Verification items for the finished model (mm, model axes). Face numbers are marked on the shaded views. A direction names the side the tool comes from. Give positions to 0.01 mm unless a question says otherwise; leave off trailing zeros. Order: outer loops, then holes, each group sorted by start corner. A loop starts at its lowest first (then second) coordinate and runs counter-clockwise, first axis right, second up. Notation, with made-up numbers: M -29,3.25 L 15,3.25 A11 ccw 15,7.25 Z; hole C 3,53.25 d4. An arc over 180 degrees is marked long. Answer as a JSON object with one key per item and string values.
```python
from build123d import *

# Parameters (mm, degrees)
CROQUIS1_W              = 100
CROQUIS1_H              = 42
SALIENTE_EXTRUIR1_DEPTH = 5
CROQUIS2_W              = 5
CROQUIS2_H              = 42
SALIENTE_EXTRUIR2_DEPTH = 38
CROQUIS3_W              = 5
CROQUIS3_H              = 42
SALIENTE_EXTRUIR3_DEPTH = 42
CROQUIS7_R              = 1.5
CORTAR_EXTRUIR1_DEPTH   = 43
CROQUIS8_R              = 12
CORTAR_EXTRUIR2_DEPTH   = 43


with BuildPart() as part:
    # Croquis1 → Saliente-Extruir1 (new body)
    with BuildSketch(Plane.XY):
        Rectangle(CROQUIS1_W, CROQUIS1_H)
        with BuildLine():
            Line((-45, 18.44), (-35.021412409, 18.44))
            ThreePointArc((-35.021412409, 18.44), (-32.021412409, 15.44), (-35.021412409, 12.44))
            Line((-35.021412409, 12.44), (-45, 12.44))
            ThreePointArc((-45, 12.44), (-48, 15.44), (-45, 18.44))
        make_face(mode=Mode.SUBTRACT)
        with BuildLine():
            Line((-45, -12.44), (-35.021412409, -12.44))
            ThreePointArc((-35.021412409, -12.44), (-32.021412409, -15.44), (-35.021412409, -18.44))
            Line((-35.021412409, -18.44), (-45, -18.44))
            ThreePointArc((-45, -18.44), (-48, -15.44), (-45, -12.44))
        make_face(mode=Mode.SUBTRACT)
    extrude(amount=SALIENTE_EXTRUIR1_DEPTH)

    # Croquis2 → Saliente-Extruir2 (add)
    with BuildSketch(Plane.XY.offset(5)):
        with Locations((47.5, 0)):
            Rectangle(CROQUIS2_W, CROQUIS2_H)
    extrude(amount=SALIENTE_EXTRUIR2_DEPTH)

    # Croquis3 → Saliente-Extruir3 (add)
    with BuildSketch(Plane.ZY.offset(-45)):
        with Locations((40.5, 0)):
            Rectangle(CROQUIS3_W, CROQUIS3_H)
    extrude(amount=SALIENTE_EXTRUIR3_DEPTH)

    # Croquis7 → Cortar-Extruir1 (cut)
    with BuildSketch(Plane.XY.offset(43)):
        with BuildLine():
            ThreePointArc((13.5, -15.5), (13.060660172, -14.439339828), (12, -14))
            Line((12, -14), (12, -15.5))
            Line((12, -15.5), (13.5, -15.5))
        make_face()
        with BuildLine():
            Line((12, -15.5), (12, -14))
            ThreePointArc((12, -14), (10.939339828, -16.560660172), (13.5, -15.5))
            Line((13.5, -15.5), (12, -15.5))
        make_face()
        with Locations((12, 15.5)):
            Circle(CROQUIS7_R)
        with Locations((43, 15.5)):
            Circle(CROQUIS7_R)
        with Locations((43, -15.5)):
            Circle(CROQUIS7_R)
    extrude(amount=-CORTAR_EXTRUIR1_DEPTH, mode=Mode.SUBTRACT)

    # Croquis8 → Cortar-Extruir2 (cut)
    with BuildSketch(Plane.XY.offset(43)):
        with Locations((27.5, 0)):
            Circle(CROQUIS8_R)
    extrude(amount=-CORTAR_EXTRUIR2_DEPTH, mode=Mode.SUBTRACT)


solid = part.part
```
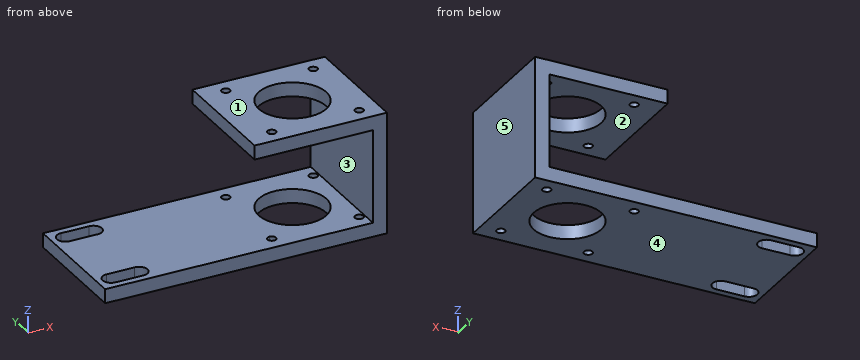
Q1. Release check for a two-part mould opening along Z. For the marked faces 3, 4 and 5 record: +Z half, -Z half, draft (parallel to the pull), parting line (faces both ways), or undercut.
Resolved:
{"face 3": "undercut", "face 4": "-Z half", "face 5": "draft"}
Q2. Gauge pin test, flat ends, axial feed: pin 1 Ø12 at (y, z) = (-13.5, 26.5) entering from -X; pin 2 Ø2.5 at (x, y) = (43, 15.5) entering from -Z; pin 3 Ø1.5 at (y, z) = (9.5, 41.5) entering from -X; pin 4 Ø8 at (x, y) = (-31.5, -1.5) entering from +Z. Record the tip position at first contact, or that the pin passes through.
Resolved:
{"pin 1": "stops at x = 45", "pin 2": "passes through", "pin 3": "stops at x = 3", "pin 4": "stops at z = 5"}
Q3. Section check C-C on x = -40.5. Record the cut outline in (y, z).
Resolved:
{"outline": "M -21,0 L -18.44,0 L -18.44,5 L -21,5 Z; M -12.44,0 L 12.44,0 L 12.44,5 L -12.44,5 Z; M 18.44,0 L 21,0 L 21,5 L 18.44,5 Z"}
Q4. Section check B-B on x = 27.5. Record the cut outline in (y, z), then the cut area to 3 significant figures.
Resolved:
{"outline": "M -21,0 L -12,0 L -12,5 L -21,5 Z; M -21,38 L -12,38 L -12,43 L -21,43 Z; M 12,0 L 21,0 L 21,5 L 12,5 Z; M 12,38 L 21,38 L 21,43 L 12,43 Z", "area": "180 mm²"}
Q5. Section check A-A on y = 0. Record the cut outline in (x, z), then the cut area to 3 significant figures.
Resolved:
{"outline": "M -50,0 L 15.5,0 L 15.5,5 L -50,5 Z; M 3,38 L 15.5,38 L 15.5,43 L 3,43 Z; M 39.5,0 L 50,0 L 50,43 L 39.5,43 L 39.5,38 L 45,38 L 45,5 L 39.5,5 Z", "area": "660 mm²"}
Q6. Tool access check on the marked faces 1 and 2. Record the directions out of +Z, -Z, +X, -X, +Y, -Y that give a thin tool (end or side, any length) a straight path to the whole face; none if there is none.
Resolved:
{"face 1": "+Z, +X, -X, +Y, -Y", "face 2": "-X, +Y, -Y"}
Q7. Section check D-D on y = 15.5. Record the cut outline in (x, z).
Resolved:
{"outline": "M -50,0 L -48,0 L -48,5 L -50,5 Z; M -32.02,0 L 10.5,0 L 10.5,5 L -32.02,5 Z; M 3,38 L 10.5,38 L 10.5,43 L 3,43 Z; M 13.5,0 L 41.5,0 L 41.5,5 L 13.5,5 Z; M 13.5,38 L 41.5,38 L 41.5,43 L 13.5,43 Z; M 44.5,0 L 50,0 L 50,43 L 44.5,43 L 44.5,38 L 45,38 L 45,5 L 44.5,5 Z"}
Q8. Material ranges on L1, parallel to Y at x = 12, z = 41.9; L2, parallel to Z at x = 36, y = 14.5; L3, parallel to X at y = 15, z = 41, recorded low to high.
Resolved:
{"L1": "y = -21 to -17, -14 to 14, 17 to 21", "L2": "z = 0 to 5, 38 to 43", "L3": "x = 3 to 10.59, 13.41 to 41.59, 44.41 to 50"}
